Work out the finished part from the listing and answer in its coordinate system (mm). Face numbers are marked on the shaded views. A direction names the side the tool comes from. Give positions to 0.01 mm unless a question says otherwise; leave off trailing zeros. Loops run counter-clockwise (first coordinate to the right, second up) from the corner with the lowest first, then second, coordinate; pieces in that order, holes last. Notation, with made-up numbers: (-3.75, -23.75) - (7.25, -23.75) arc R17 cw to (7.25, 5.25) - close; hole circle Ø6 at (-16, 16.5). An arc over 180 degrees is marked (long way). One line per item, written item: value.
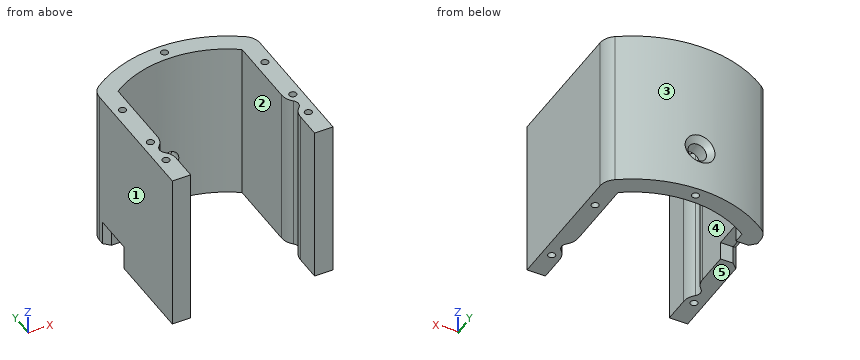
Autodesk Inventor part; units mm, degrees
ref_plane "YZ Plane" through (0, 0, 0) normal (1, 0, 0) x (0, 1, 0)
ref_plane "XZ Plane" through (0, 0, 0) normal (0, 1, 0) x (-1, 0, 0)
ref_plane "XY Plane" through (0, 0, 0) normal (0, 0, 1) x (1, 0, 0)
sketch "Sketch1" plane through (0, 0, 0) normal (0, 0, 1) x (1, 0, 0)
  arc A0 (40.4395, 56.9532) -> (-40.4395, 56.9532) centre (0, 0) ccw
  arc A1 (-40.4395, 56.9532) -> (-44.45, 49.1869) centre (-34.925, 49.1869) ccw
  circle A2 centre (0, 64.77) radius 2
  arc A3 (44.45, 49.1869) -> (40.4395, 56.9532) centre (34.925, 49.1869) ccw
  line L0 (44.45, -25.4935) -> (44.45, 49.1869)
  line L1 (-44.45, 49.1869) -> (-44.45, -25.4935)
  circle A4 centre (-39.37, 34.8315) radius 2
  circle A5 centre (39.37, 34.8315) radius 2
  circle A6 centre (39.37, -9.6185) radius 2
  circle A7 centre (-39.37, -9.6185) radius 2
  circle A8 centre (-34.6, -1.2888) radius 2
  circle A9 centre (34.6, -1.2888) radius 2
  line L2 (-39.37, -9.6185) -> (-39.37, -25.4935)
  line L3 (-39.37, -25.4935) -> (-44.45, -25.4935)
  circle A10 centre (-34.6, -1.2888) radius 3.81
  circle A11 centre (34.6, -1.2888) radius 3.81
  line L4 (-34.29, -25.4935) -> (-34.29, 48.8579)
  arc A12 (34.29, 48.8579) -> (-34.29, 48.8579) centre (0, 0) ccw
  line L5 (34.29, 48.8579) -> (34.29, -25.4935)
  line L6 (-39.37, -25.4935) -> (-34.29, -25.4935)
  line L7 (34.29, -25.4935) -> (44.45, -25.4935)
  point P0 (0, 0)
  point P1 (-34.29, -5.0862)
  point P2 (-34.29, 2.5086)
  point P3 (34.29, 2.5086)
  point P4 (34.29, -5.0862)
  dimension "d0" = 7.62
  dimension "d1" = 7.62
  dimension "d2" = 10.16
extrude "Extrusion1" add sketch "Sketch1" along normal blind 88.9 contours A3 L0 L7 L5 A11 A12 L4 A10 L6 L3 L1 A1 A0 | A2 | A4
fillet "Fillet1" radius 9.525 4 edges at (-34.29, 2.5086, 44.45) (34.29, 2.5086, 44.45) (-34.29, -5.0862, 44.45) (34.29, -5.0862, 44.45)
sketch "Sketch5" plane through (34.29, -25.4935, 0) normal (0, -1, 0) x (1, 0, 0)
  line L0 (-68.58, 0) -> (-68.58, 88.9)
  line L1 (0, 88.9) -> (0, 0)
  line L2 (-68.58, 0) -> (0, 0)
  line L3 (-68.58, 0) -> (-34.29, 0)
  line L4 (-34.29, 0) -> (-34.29, 88.9)
  line L5 (-34.29, 0) -> (-34.29, 25.4)
  circle A0 centre (-34.29, 25.4) radius 5.08
  dimension "d39" = 25.4
  dimension "d40" = 10.16
extrude "Extrusion5" cut sketch "Sketch5" against normal through all
sketch "Sketch6" plane through (0, 0, 0) normal (0, 0, -1) x (-1, 0, 0)
  arc A0 (-34.29, -10.9276) -> (-37.2329, -4.0427) centre (-43.815, -10.9276) ccw
  arc A1 (-37.2329, 1.4651) -> (-37.2329, -4.0427) centre (-34.6, -1.2888) ccw
  arc A2 (-37.2329, 1.4651) -> (-34.29, 8.35) centre (-43.815, 8.35) ccw
  line L0 (-34.29, 48.8579) -> (-34.29, 8.35)
  arc A3 (34.29, 48.8579) -> (-34.29, 48.8579) centre (0, 0) ccw
  line L1 (34.29, 8.35) -> (34.29, 48.8579)
  arc A4 (34.29, 8.35) -> (37.2329, 1.4651) centre (43.815, 8.35) ccw
  arc A5 (37.2329, -4.0427) -> (37.2329, 1.4651) centre (34.6, -1.2888) ccw
  arc A6 (37.2329, -4.0427) -> (34.29, -10.9276) centre (43.815, -10.9276) ccw
  line L2 (34.29, -25.4935) -> (34.29, -10.9276)
  line L3 (44.45, -25.4935) -> (34.29, -25.4935)
  line L4 (44.45, 49.1869) -> (44.45, -25.4935)
  arc A7 (44.45, 49.1869) -> (40.4395, 56.9532) centre (34.925, 49.1869) ccw
  arc A8 (40.4395, 56.9532) -> (-40.4395, 56.9532) centre (0, 0) ccw
  arc A9 (-40.4395, 56.9532) -> (-44.45, 49.1869) centre (-34.925, 49.1869) ccw
  line L5 (-44.45, -25.4935) -> (-44.45, 49.1869)
  line L6 (-34.29, -25.4935) -> (-44.45, -25.4935)
  line L7 (-34.29, -10.9276) -> (-34.29, -25.4935)
  circle A10 centre (39.37, -9.6185) radius 2
  circle A11 centre (-39.37, -9.6185) radius 2
  circle A12 centre (-39.37, 34.8315) radius 2
  line L8 (39.37, 34.8315) -> (39.37, 42.769)
  line L9 (39.37, 42.769) -> (39.37, 26.894)
  line L10 (39.37, 42.769) -> (47.6019, 42.769)
  line L11 (39.37, 26.894) -> (47.6019, 26.894)
  line L12 (39.37, 42.769) -> (31.4554, 42.769)
  line L13 (39.37, 26.894) -> (31.1414, 26.894)
  point P0 (0, 0)
  point P1 (34.29, 42.769)
  point P2 (34.29, 26.894)
  point P3 (44.45, 26.894)
  point P4 (44.45, 42.769)
  dimension "d43" = 7.9375
  dimension "d44" = 15.875
extrude "Extrusion6" cut sketch "Sketch6" against normal blind 10.16 contours L12 L8 L9 L13 L1 | L10 L4 L11 L9 L8
chamfer "Chamfer3" distance 3.175 angle 45 3 edges at (-44.45, 34.8315, 10.16) (-44.45, 42.769, 5.08) (-44.45, 26.894, 5.08)
chamfer "Chamfer4" distance 3.175 angle 45 1 edges at (-5.0799, 69.665, 25.4351)
sketch "Sketch7" plane through (0, 0, 88.9) normal (0, 0, 1) x (1, 0, 0)
  circle A0 centre (0, 64.77) radius 2
  circle A1 centre (-39.37, 34.8315) radius 2
  point P0 (0, 0)
extrude "Extrusion7" cut sketch "Sketch7" against normal blind 25.4
sketch "Sketch8" plane through (0, 0, 0) normal (0, 0, -1) x (-1, 0, 0)
  point P0 (0, 0)
extrude "Extrusion8" cut sketch "Sketch1" along normal blind 15.24 contours A2
sketch "Sketch9" plane through (0, 0, 88.9) normal (0, 0, 1) x (1, 0, 0)
  circle A0 centre (-39.37, 34.8315) radius 2
  line L0 (-39.37, 34.8315) -> (-39.37, 6.2565)
  circle A1 centre (-39.37, 6.2565) radius 2
  circle A2 centre (39.37, 34.8315) radius 2
  line L1 (39.37, 34.8315) -> (39.37, 6.2565)
  circle A3 centre (39.37, 6.2565) radius 2
  point P0 (0, 0)
  dimension "d57" = 28.575
  dimension "d58" = 4
  dimension "d59" = 28.575
  dimension "d60" = 4
extrude "Extrusion9" cut sketch "Sketch9" against normal blind 15.24 contours A1 | A3
properties part number "back wall"
1. For the marked faces 4 and 5, determine the directions among +Z, -Z, +X, -X, +Y, -Y from which every point of the face is accessible in a straight line to the end or side of a thin tool.
Output:
face 4: +Z, -Z, -Y
face 5: -Z, +X, -X, +Y, -Y
2. The mould has two halves that part along X. Classify the marked faces 1, 2 and 3: released by +X, released by -X, zero draft, split by the parting line, or undercut.
Output:
face 1: released by -X
face 2: undercut
face 3: split by the parting line
3. Flat-ended cylindrical pins translate along their axes: pin 1 Ø4.5 at (x, y) = (-39.37, 34.83) entering from -Z; pin 2 Ø8 at (x, z) = (9, 22) entering from +Y; pin 3 Ø2 at (x, z) = (33.5, 51) entering from +Y. Find the tip coordinate at first contact, or state that the pin passes through.
Output:
pin 1: stops at z = 10.16
pin 2: stops at y = 69.61
pin 3: stops at y = 61.83
4. Section C-C (y = 64.77) is taken. Write down the section's boundary in (x, z), and give its area (3 significant figures).
Output:
outline: (-26.15, 0) - (-2, 0) - (-2, 15.24) - (2, 15.24) - (2, 0) - (26.15, 0) - (26.15, 88.9) - (2, 88.9) - (2, 63.5) - (-2, 63.5) - (-2, 88.9) - (-26.15, 88.9) - close; hole circle Ø10.16 at (0, 25.4)
area: 4,410 mm²
5. Section B-B (z = 47) is taken. Count the separate pieces of the cut face and the enclosed holes in it, and give its area (3 significant figures).
Output:
separate pieces: 1
enclosed holes: 3
area: 2,310 mm²
6. Find the intervals of material crossed by line 1 along X through (y, z) = (20.5, 13); line 2 along Y through (x, z) = (39.5, 31); line 3 along Y through (x, z) = (39, 80), in increasing order.
Output:
line 1: x = -44.45 to -34.29, 34.29 to 44.45
line 2: y = -25.49 to -11.61, -7.62 to 32.84, 36.83 to 57.61
line 3: y = -25.49 to -11.58, -7.65 to 4.29, 8.22 to 32.87, 36.8 to 57.95
7. Section A-A (y = -13) is taken. Write down the section's boundary in (x, z), and give its area (3 significant figures).
Output:
outline: (-44.45, 0) - (-34.29, 0) - (-34.29, 88.9) - (-44.45, 88.9) - close; (34.29, 0) - (44.45, 0) - (44.45, 88.9) - (34.29, 88.9) - close
area: 1,810 mm²
